Can you work these out from the model? Positions are in its coordinate system, mm. Round coordinates to 2 decimals unless told otherwise and drop trailing zeros. Order: outer loops, then holes, each group sorted by start corner. A loop starts at its lowest first (then second) coordinate and runs counter-clockwise, first axis right, second up. Notation, with made-up numbers: (69.25, 19.5) - (114.25, 19.5) arc R25 cw to (114.25, 54.5) - close; hole circle Ø6 at (-20, 21.25). An arc over 180 degrees is marked (long way). Write item = value, one per line.
Autodesk Inventor part; units mm, degrees
ref_plane "Start Plane" through (0, 0, -9.7188) normal (0, 0, 1) x (1, 0, 0)
ref_plane "End Plane" through (0, 0, 148.8552) normal (0, 0, 1) x (1, 0, 0)
ref_plane "Work Plane4" through (2.3525, 9.2299, -7.9924) normal (-0.1588, -0.6229, -0.766) x (0.8923, -0.4227, 0.1588)
ref_plane "Start Plane" through (0, 0, -9.7188) normal (0, 0, 1) x (1, 0, 0)
ref_plane "End Plane" through (0, 0, 148.8552) normal (0, 0, 1) x (1, 0, 0)
sketch "Sketch" plane through (0, 0, 0) normal (0, 0, 1) x (1, 0, 0)
  circle A0 centre (0, 0) radius 9.525
  dimension "d0" = 19.05
extrude "Body" add sketch "Sketch" along normal up to surface (158.574 mm away) from surface at -9.7188
sketch "Sketch2" plane through (0, 0, 0) normal (0, 0, 1) x (1, 0, 0)
  line L0 (0, 0) -> (10, 0)
ref_plane "Work Plane3" through (0, 0, 0) normal (0, -1, 0) x (1, 0, 0)
ref_plane "Work Plane4" through (2.3525, 9.2299, -7.9924) normal (-0.1588, -0.6229, -0.766) x (0.8923, -0.4227, 0.1588)
split "Split1" plane through (2.3525, 9.2299, -7.9924) removes the side toward (-0.1588, -0.6229, -0.766)
ref_plane "Work Plane5" through (2.3525, 9.2299, 146.4032) normal (-0.1892, -0.7423, 0.6428) x (0.9782, -0.0855, 0.1892)
split "Split2" plane through (2.3525, 9.2299, 146.4032) removes the side toward (-0.1892, -0.7423, 0.6428)
sketch "Sketch3" plane through (0, 0, 0) normal (0, -1, 0) x (1, 0, 0)
  line L0 (-2, -9.7188) -> (12, -9.7188)
  line L1 (-2, 148.8552) -> (12, 148.8552)
  dimension "d7" = 158.574
equation "\"d0\" = Diam"
equation "\"d1\" = G_L"
equation "\"Diam\" = 19.05"
equation "\"G_L\" = 154.39562"
equation "\"G_OFFSET_START\" = 9.71882"
equation "\"G_OFFSET_END\" = 13.80341"
equation "\"d4\" = -G_OFFSET_START"
equation "\"d5\" = G_OFFSET_END + B_L"
equation "\"B_L\" = 135.05174"
properties part number "ANSI/AISC Rolled Steel - 3/4-6.079, RB" material "Steel, Mild"
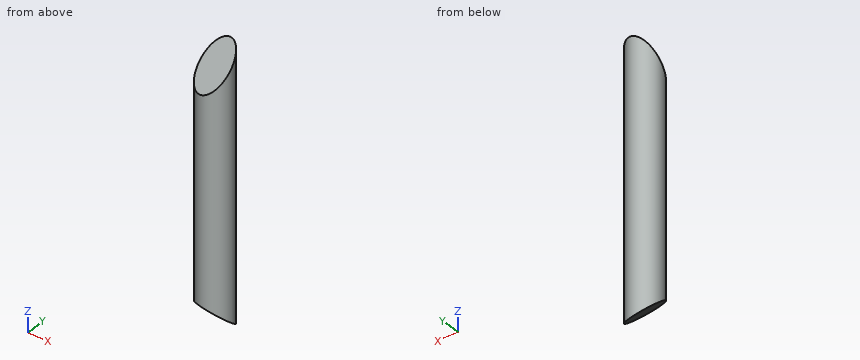
(1) If we section it at B-B (y = -6.5): Write out the boundary of the cut face in (x, z).
Computed:
outline = (-6.96, 6.73) - (6.96, 3.84) - (6.96, 129.6) - (-6.96, 125.5) - close
(2) Will these pins go through, and if not, where does the flat tip stop? P1, Ø1.5, axis at x = -3, y = -1, coming from the -Z side; P2, Ø1.5, axis at x = 5, z = 24, coming from the -Y side; P3, Ø1.5, axis at x = -3, y = 0, coming from the -Z side; P4, Ø2, axis at x = -1, z = 50.5, coming from the -Y side (3 decimals).
Computed:
P1 = 0.81
P2 = -8.52
P3 = -0.01
P4 = -9.525
(3) If I drill on line 1 (X direction, y = 0.75, z = 25); line 2 (Y direction, x = 0.5, z = 53.5); line 3 (X direction, y = 3, z = 71.5), over which ranges is the centre line in solid material (lowest first)? Write a range as from..to.
Computed:
line_1 = -9.5..9.5
line_2 = -9.51..9.51
line_3 = -9.04..9.04
(4) If we section it at C-C (x = 8): Write out the boundary of the cut face in (y, z), plus the area to 3 significant figures.
Computed:
outline = (-5.17, 2.55) - (5.17, -5.86) - (5.17, 143.38) - (-5.17, 131.44) - close
area = 1,440 mm^2
(5) If we section it at D-D (z = 133.5): Write out the boundary of the cut face in (x, y) (3 decimals).
Computed:
outline = (-9.465, 1.068) - (8.822, -3.593) arc R9.525 ccw (long way) to start
(6) If we section it at A-A (z = 47.5): Write out the boundary of the cut face in (x, y) (3 decimals).
Computed:
outline = circle Ø19.05 at (0, 0)
